```python
from build123d import *

# Parameters (mm, degrees)
SKETCH1_R           = 7.62
BOSS_EXTRUDE1_DEPTH = 3.175
SKETCH3_R           = 0.508
CUT_EXTRUDE1_DEPTH  = 25.4
SKETCH6_W           = 1.220456994
SKETCH6_H           = 1.016
CUT_EXTRUDE2_DEPTH  = 7.366
SKETCH7_W           = 1.220456994
SKETCH7_H           = 1.016
CUT_EXTRUDE3_DEPTH  = 7.366
SKETCH4_R           = 0.508


with BuildPart() as part:
    # Sketch1 → Boss-Extrude1 (new body)
    with BuildSketch(Plane(origin=(0, 0, 0), x_dir=(1, 0, 0), z_dir=(0, 1, 0))):
        Circle(SKETCH1_R)
    extrude(amount=BOSS_EXTRUDE1_DEPTH)

    # Sketch3 → Cut-Extrude1 (cut, symmetric)
    with BuildSketch(Plane.XY):
        with Locations((-6.604, 1.5875)):
            Circle(SKETCH3_R)
    extrude(amount=CUT_EXTRUDE1_DEPTH, both=True, mode=Mode.SUBTRACT)

    # Sketch6 → Cut-Extrude2 (cut)
    with BuildSketch(Plane.XY.offset(-7.62)):
        with Locations((-7.214228497, 1.5875)):
            Rectangle(SKETCH6_W, SKETCH6_H)
    extrude(amount=CUT_EXTRUDE2_DEPTH, mode=Mode.SUBTRACT)

    # Sketch7 → Cut-Extrude3 (cut)
    with BuildSketch(Plane.XY.offset(7.62)):
        with Locations((-7.214228497, 1.5875)):
            Rectangle(SKETCH7_W, SKETCH7_H)
    extrude(amount=-CUT_EXTRUDE3_DEPTH, mode=Mode.SUBTRACT)

    # Cut-Sweep1: sweep along a path in Sketch5
    with BuildLine(Plane(origin=(0, 0, 0), x_dir=(1, 0, 0), z_dir=(0, 1, 0))) as cut_sweep1_path:
        ThreePointArc((-7.554809844, -0.994609585), (7.62, 0), (-7.554809844, 0.994609585))
    # Sketch4 → Cut-Sweep1 (sweep, cut)
    with BuildSketch(Plane.XY):
        with Locations((7.62, 1.5875)):
            Circle(SKETCH4_R)
    sweep(path=cut_sweep1_path.line, mode=Mode.SUBTRACT)


solid = part.part
```
Model file for the job. Use its own axes, mm. A direction names the side the tool comes from. Coordinates: 2 decimals unless noted, no trailing zeros. Order: outer loops, then holes, each group sorted by start corner. A loop starts at its lowest first (then second) coordinate and runs counter-clockwise, first axis right, second up. Notation, with made-up numbers: (34.5, 71) - (49.5, 71) arc R24 cw to (49.5, 108) - close; hole circle Ø4 at (34, 56.25). An arc over 180 degrees is marked (long way). Return JSON: item names as keys, results as strings. Group by question number.
1) Probe line 1 (Y direction, x = 4.5, z = -5.75) (3 decimals); line 2 (Y direction, x = 2.5, z = 7) (3 decimals); line 3 (X direction, y = 0.5, z = -3.5). List the from-to ranges inside material, lowest first. Write a range as from..to.
2) Tool access for faces 4 (the flat face through (0, 0, 0)), 5 (the flat face through (-7.3, 1.6, 0.254)), 6 (the flat face through (-7, 2.096, -2)): list every direction of +Z, -Z, +X, -X, +Y, -Y with a clear straight run to the whole face (end or side of a thin tool).
3) Mould opens along X. For faces 1 (the cylindrical face through (-6.135, 1.393, 0.053)), 2 (the flat face through (-7, 1.08, 2)), 3 (the cylindrical face through (3.52, 0.86, 6.76)) say: released by +X, released by -X, zero draft, split by the parting line, or undercut.
4) Saw through at A-A, the plane z = 0. Write the cut outline in (x, y) (1 decimal), plus the area to 3 significant figures.
5) Saw through at B-B, the plane y = 0.25. Write the cut outline in (x, z), plus the area to 3 significant figures.
6) Flat gauge pins, fed straight in: P1, Ø1, axis at x = 1, y = 2, coming from the -Z side; P2, Ø0.5, axis at x = -7.5, z = 3, coming from the -Y side; P3, Ø1, axis at y = 3, z = 2, coming from the -X side; P4, Ø0.5, axis at x = -7, y = 1.5, coming from the -Z side. Where does each tip first touch, or does it go through?
Values found:
{
 "1": {"line 1": "y = 0..1.192, 1.983..3.175", "line 2": "y = 0..1.115, 2.06..3.175", "line 3": "x = -6.77..6.77"},
 "2": {"face 4": "+Z, -Z, +X, -X, -Y", "face 5": "+Z, -X", "face 6": "-Z, -X"},
 "3": {"face 1": "undercut", "face 2": "zero draft", "face 3": "split by the parting line"},
 "4": {"outline": "(-7.6, 0) - (7.6, 0) - (7.6, 1.1) arc R0.5 cw to (7.6, 2.1) - (7.6, 3.2) - (-7.6, 3.2) - close; hole circle Ø1 at (-6.6, 1.6)", "area": "47.2 mm²"},
 "5": {"outline": "circle Ø15.24 at (0, 0)", "area": "182 mm²"},
 "6": {"P1": "stops at z = -7.6", "P2": "passes through", "P3": "stops at x = -7.47", "P4": "stops at z = -0.25"}
}
